Could you check a few things on this model? Use its own coordinates, in mm. Give positions to 0.01 mm unless a question says otherwise; leave off trailing zeros. Loops run counter-clockwise (first coordinate to the right, second up) from the corner with the lowest first, then second, coordinate; pieces in that order, holes last. Notation, with made-up numbers: M 45.25,-10 L 93.25,-10 A15 cw 93.25,14 Z; hole C 50.25,20 d4. An arc over 180 degrees is marked long. Return JSON: item names as keys, results as strings. Group by question number.
1. If we section it at B-B (z = -16.5): Write out the boundary of the cut face in (x, y), plus the area to 3 significant figures.
2. For pin 1 (1 mm diameter, centred on x = 1, z = 8, fed in from -Y); pin 2 (1 mm diameter, centred on x = 1, z = 1.5, fed in from +Y), each with a flat end and sliding along its axis, tell me the tip position at first contact or that it passes through.
3. If we section it at C-C (z = 75): Write out the boundary of the cut face in (x, y), plus the area to 3 significant figures.
4. If we section it at A-A (y = -102): Write out the boundary of the cut face in (x, z).
5. If we section it at D-D (x = 1.2): State how many separate pieces and enclosed holes the cut face has, plus the area to 3 significant figures.
6. Please list where these lines run through material, in increasing order: line 1 (Y direction, x = 1.5, z = -97.5); line 2 (Y direction, x = 0.5, z = -100.35); line 3 (Y direction, x = 1.05, z = 53.45).
Autodesk Inventor part; units mm, degrees
ref_plane "YZ Plane" through (0, 0, 0) normal (1, 0, 0) x (0, 1, 0)
ref_plane "XZ Plane" through (0, 0, 0) normal (0, 1, 0) x (-1, 0, 0)
ref_plane "XY Plane" through (0, 0, 0) normal (0, 0, 1) x (1, 0, 0)
sketch "Sketch2" plane through (0, 0, 0) normal (1, 0, 0) x (0, 1, 0)
  line L0 (-123.2, 103.45) -> (123.2, 103.45)
  line L1 (123.2, 103.45) -> (123.2, -103.45)
  line L2 (123.2, -103.45) -> (-123.2, -103.45)
  line L3 (-123.2, -103.45) -> (-123.2, 103.45)
  line L4 (-123.2, 103.45) -> (123.2, -103.45) construction
  line L5 (123.2, 103.45) -> (-123.2, -103.45) construction
  point P0 (0, 0)
  dimension "d4" = 246.4
  dimension "d5" = 206.9
extrude "Extrusion2" add sketch "Sketch2" along normal blind 2
sketch "Sketch3" plane through (2, 0, 0) normal (1, 0, 0) x (0, 0, -1)
  line L0 (103.45, 123.2) -> (-103.45, 123.2) construction
  line L1 (-103.45, -123.2) -> (103.45, -123.2) construction
  line L2 (-103.45, 123.2) -> (-103.45, -123.2) construction
  line L3 (-53.45, 37.85) -> (-53.45, -37.35) construction
  line L4 (-23.45, -123.2) -> (-23.45, 123.2) construction
  point P0 (0, 0)
  point P1 (-23.45, 70.45)
  point P2 (-23.45, 57.85)
  point P3 (-53.45, 25.25)
  point P4 (-53.45, -24.75)
  point P5 (-23.45, -57.35)
  point P6 (-23.45, -69.95)
  dimension "d8" = 12.6
  dimension "d9" = 12.6
  dimension "d10" = 12.6
  dimension "d11" = 12.6
  dimension "d15" = 53.25
  dimension "d24" = 50
  dimension "d25" = 80
  dimension "d26" = 0
  dimension "d27" = 0
  dimension "d28" = 20
  dimension "d29" = 50
  dimension "d30" = 20
hole "mounting of front power splitters" at (2, 70.45, 23.45) at (2, 57.85, 23.45) at (2, 37.85, 53.45) at (2, 25.25, 53.45) at (2, -24.75, 53.45) at (2, -37.35, 53.45) at (2, -57.35, 23.45) at (2, -69.95, 23.45) direction (-1, 0, 0) diameter 2.013 end through all
sketch "Sketch4" plane through (2, 0, 0) normal (1, 0, 0) x (0, 0, -1)
  line L0 (-103.45, 123.2) -> (-103.45, -123.2) construction
  line L1 (-103.45, -56.5) -> (103.45, -56.5) construction
  line L2 (103.45, -123.2) -> (103.45, 123.2) construction
  line L3 (-103.45, -23.9) -> (103.45, -23.9) construction
  line L4 (-103.45, 38.7) -> (103.45, 38.7) construction
  line L5 (-103.45, 71.3) -> (103.45, 71.3) construction
  line L6 (-103.45, -123.2) -> (103.45, -123.2) construction
  point P0 (0, 0)
  point P1 (100.35, -56.5)
  point P2 (87.75, -56.5)
  point P3 (70.35, -23.9)
  point P4 (57.75, -23.9)
  point P5 (70.35, 38.7)
  point P6 (57.75, 38.7)
  point P7 (100.35, 71.3)
  point P8 (87.75, 71.3)
  dimension "d32" = 66.7
  dimension "d33" = 32.6
  dimension "d34" = 62.6
  dimension "d35" = 32.6
  dimension "d36" = 12.6
  dimension "d37" = 12.6
  dimension "d38" = 12.6
  dimension "d39" = 12.6
  dimension "d40" = 3.1
  dimension "d41" = 33.1
  dimension "d42" = 33.1
  dimension "d43" = 3.1
hole "mounting of rear power splitters" at (2, -56.5, -100.35) at (2, -56.5, -87.75) at (2, -23.9, -70.35) at (2, -23.9, -57.75) at (2, 38.7, -70.35) at (2, 38.7, -57.75) at (2, 71.3, -100.35) at (2, 71.3, -87.75) direction (-1, 0, 0) diameter 2.013 end through all
sketch "Sketch5" plane through (2, 0, 0) normal (1, 0, 0) x (0, 0, -1)
  line L0 (-103.45, -123.2) -> (103.45, -123.2)
  line L1 (-87.25, -83.2) -> (87.25, -83.2)
  line L2 (87.25, -83.2) -> (87.25, -123.2)
  line L3 (87.25, -123.2) -> (-87.25, -123.2)
  line L4 (-87.25, -123.2) -> (-87.25, -83.2)
  line L5 (-87.25, -83.2) -> (87.25, -123.2) construction
  line L6 (87.25, -83.2) -> (-87.25, -123.2) construction
  line L7 (-103.45, 123.2) -> (-103.45, -123.2)
  line L8 (103.45, -123.2) -> (103.45, 123.2)
  line L9 (-87.25, 83.2) -> (87.25, 83.2)
  line L10 (87.25, 83.2) -> (87.25, 123.2)
  line L11 (87.25, 123.2) -> (-87.25, 123.2)
  line L12 (-87.25, 123.2) -> (-87.25, 83.2)
  line L13 (-87.25, 83.2) -> (87.25, 123.2) construction
  line L14 (87.25, 83.2) -> (-87.25, 123.2) construction
  line L15 (103.45, 123.2) -> (-103.45, 123.2)
  point P0 (0, 0)
  point P1 (0, -103.2)
  point P2 (0, 103.2)
  point P3 (87.25, 103.2)
  point P4 (-87.25, -123.2)
  dimension "d51" = 16.2
  dimension "d52" = 16.2
  dimension "d53" = 40
  dimension "d54" = 16.2
  dimension "d55" = 16.2
  dimension "d56" = 40
  dimension "d57" = 0
extrude "Extrusion3" cut sketch "Sketch5" against normal blind 2 contours L4 L1 L2 L0 | L11 L10 L9 L12
sketch "Sketch6" plane through (2, 0, 0) normal (1, 0, 0) x (0, 0, -1)
  line L0 (-50.35, 54.25) -> (54.65, 54.25)
  line L1 (54.65, 54.25) -> (54.65, -54.75)
  line L2 (54.65, -54.75) -> (-50.35, -54.75)
  line L3 (-50.35, -54.75) -> (-50.35, 54.25)
  line L4 (103.45, -123.2) -> (103.45, 123.2)
  line L5 (103.45, 123.2) -> (87.25, 123.2)
  point P0 (0, 0)
  dimension "d60" = 105
  dimension "d61" = 109
  dimension "d62" = 48.8
  dimension "d63" = 68.95
extrude "Extrusion4" cut sketch "Sketch6" against normal blind 2
sketch "Sketch7" plane through (2, 0, 0) normal (1, 0, 0) x (0, 0, -1)
  line L0 (87.25, -123.2) -> (103.45, -123.2) construction
  line L1 (97.5, -123.2) -> (97.5, 123.2) construction
  line L2 (103.45, 123.2) -> (87.25, 123.2) construction
  line L3 (103.45, -123.2) -> (103.45, 123.2) construction
  line L4 (-87.25, 123.2) -> (-103.45, 123.2) construction
  line L5 (-97.5, 123.2) -> (-97.5, -123.45) construction
  line L6 (-103.45, 123.2) -> (-103.45, -123.2) construction
  line L7 (-103.45, -123.2) -> (-87.25, -123.2) construction
  point P0 (0, 0)
  point P1 (-97.5, -117.2)
  point P2 (-97.5, -111.2)
  point P3 (97.5, -117.2)
  point P4 (97.5, -111.2)
  point P5 (-97.5, 117.2)
  point P6 (-97.5, 111.2)
  point P7 (97.5, 117.2)
  point P8 (97.5, 111.2)
  point P9 (-87.25, -123.2)
  dimension "d66" = 5.95
  dimension "d67" = 5.95
  dimension "d68" = 6
  dimension "d69" = 6
  dimension "d70" = 6
  dimension "d71" = 6
  dimension "d72" = 6
  dimension "d73" = 6
  dimension "d74" = 6
  dimension "d75" = 6
hole "Hole3" at (2, -117.2, 97.5) at (2, -111.2, 97.5) at (2, -117.2, -97.5) at (2, -111.2, -97.5) at (2, 117.2, 97.5) at (2, 111.2, 97.5) at (2, 117.2, -97.5) at (2, 111.2, -97.5) direction (-1, 0, 0) diameter 2.013 end through all
sketch "DFX Export" plane through (2, 0, 0) normal (1, 0, 0) x (0, 0, -1)
  line L0 (-103.45, 123.2) -> (-103.45, -123.2)
  line L1 (-103.45, 123.2) -> (-103.45, -123.2)
  line L2 (-87.25, -123.2) -> (-87.25, -83.2)
  line L3 (-103.45, -123.2) -> (-87.25, -123.2)
  line L4 (-87.25, -123.2) -> (-87.25, -83.2)
  line L5 (87.25, -123.2) -> (87.25, -83.2)
  line L6 (-87.25, -83.2) -> (87.25, -83.2)
  line L7 (87.25, -83.2) -> (87.25, -123.2)
  line L8 (87.25, -123.2) -> (103.45, -123.2)
  line L9 (87.25, -123.2) -> (103.45, -123.2)
  line L10 (103.45, 123.2) -> (87.25, 123.2)
  line L11 (103.45, -123.2) -> (103.45, 123.2)
  line L12 (103.45, 123.2) -> (87.25, 123.2)
  line L13 (87.25, 83.2) -> (-87.25, 83.2)
  line L14 (87.25, 123.2) -> (87.25, 83.2)
  line L15 (87.25, 83.2) -> (-87.25, 83.2)
  line L16 (-87.25, 123.2) -> (-103.45, 123.2)
  line L17 (-87.25, 83.2) -> (-87.25, 123.2)
  line L18 (-87.25, 123.2) -> (-103.45, 123.2)
  point P0 (0, 0)
properties part number "mounting-plate"
Answer:
{
 "1": {"outline": "M 0,-83.2 L 2,-83.2 L 2,-54.75 L 0,-54.75 Z; M 0,54.25 L 2,54.25 L 2,83.2 L 0,83.2 Z", "area": "115 mm²"},
 "2": {"pin 1": "stops at y = -83.2", "pin 2": "stops at y = 83.2"},
 "3": {"outline": "M 0,-83.2 L 2,-83.2 L 2,83.2 L 0,83.2 Z", "area": "333 mm²"},
 "4": {"outline": "M 0,-103.45 L 2,-103.45 L 2,-87.25 L 0,-87.25 Z; M 0,87.25 L 2,87.25 L 2,103.45 L 0,103.45 Z"},
 "5": {"separate pieces": "1", "enclosed holes": "25", "area": "25,500 mm²"},
 "6": {"line 1": "y = -123.2 to -118.21, -116.19 to -112.21, -110.19 to 110.19, 112.21 to 116.19, 118.21 to 123.2", "line 2": "y = -123.2 to -57.51, -55.49 to 70.29, 72.31 to 123.2", "line 3": "y = -83.2 to -38.36, -36.34 to -25.76, -23.74 to 24.24, 26.26 to 36.84, 38.86 to 83.2"}
}
